```python
from build123d import *

# Parameters (mm, degrees)
F1_DEPTH = 25.4
F3_DEPTH = 25.401
F5_DEPTH = 25.401


with BuildPart() as f1:
    # F0 (on Top) → F1 (new body)
    with BuildSketch(Plane.XY):
        with BuildLine():
            Line((58.851477, 66.675), (0, 66.675))
            Line((0, 66.675), (-69.85, 66.675))
            Line((-69.85, 66.675), (-69.85, 53.975))
            ThreePointArc((-69.85, 53.975), (-71.709872, 49.484872), (-76.2, 47.625))
            Line((-76.2, 47.625), (-88.9, 47.625))
            ThreePointArc((-88.9, 47.625), (-93.390128, 45.765128), (-95.25, 41.275))
            Line((-95.25, 41.275), (-95.25, -79.375))
            ThreePointArc((-95.25, -79.375), (-93.390128, -83.865128), (-88.9, -85.725))
            Line((-88.9, -85.725), (-76.2, -85.725))
            ThreePointArc((-76.2, -85.725), (-71.709872, -83.865128), (-69.85, -79.375))
            Line((-69.85, -79.375), (-69.85, -73.025))
            ThreePointArc((-69.85, -73.025), (-67.990128, -68.534872), (-63.5, -66.675))
            Line((-63.5, -66.675), (0, -66.675))
            Line((0, -66.675), (63.5, -66.675))
            ThreePointArc((63.5, -66.675), (67.990128, -68.534872), (69.85, -73.025))
            Line((69.85, -73.025), (69.85, -79.375))
            ThreePointArc((69.85, -79.375), (71.709872, -83.865128), (76.2, -85.725))
            Line((76.2, -85.725), (88.9, -85.725))
            ThreePointArc((88.9, -85.725), (93.390128, -83.865128), (95.25, -79.375))
            Line((95.25, -79.375), (95.25, 41.275))
            ThreePointArc((95.25, 41.275), (93.390128, 45.765128), (88.9, 47.625))
            Line((88.9, 47.625), (73.516174, 47.625))
            ThreePointArc((73.516174, 47.625), (70.341174, 48.475739), (68.016913, 50.8))
            Line((68.016913, 50.8), (58.851477, 66.675))
        make_face()
        with BuildLine():
            ThreePointArc((-85.725, 31.75), (-82.55, 34.925), (-79.375, 31.75))
            Line((-79.375, 31.75), (-79.375, -69.85))
            ThreePointArc((-79.375, -69.85), (-82.55, -73.025), (-85.725, -69.85))
            Line((-85.725, -69.85), (-85.725, 31.75))
        make_face(mode=Mode.SUBTRACT)
        with BuildLine():
            Line((79.375, -69.85), (79.375, 31.75))
            ThreePointArc((79.375, 31.75), (82.55, 34.925), (85.725, 31.75))
            Line((85.725, 31.75), (85.725, -69.85))
            ThreePointArc((85.725, -69.85), (82.55, -73.025), (79.375, -69.85))
        make_face(mode=Mode.SUBTRACT)
    extrude(amount=F1_DEPTH)

    # F2 (on face) → F3 (cut, through all)
    with BuildSketch(Plane.XY.offset(25.4)):
        Polygon((65.975549, 43.337223), (52.501477, 66.675), (47.738977, 66.675), (62.403674, 41.275), align=None)
    extrude(amount=-F3_DEPTH, mode=Mode.SUBTRACT)

    # F4 (on face) → F5 (cut, through all)
    with BuildSketch(Plane.XY.offset(25.4)):
        Polygon((62.195398, 30.637223), (41.388977, 66.675), (36.626477, 66.675), (58.623523, 28.575), align=None)
        Polygon((62.08142, 11.587223), (30.276477, 66.675), (25.513977, 66.675), (58.509545, 9.525), align=None)
        Polygon((19.163977, 66.675), (14.401477, 66.675), (47.397045, 9.525), (50.96892, 11.587223), align=None)
        Polygon((8.051477, 66.675), (3.288977, 66.675), (36.284545, 9.525), (39.85642, 11.587223), align=None)
        Polygon((-3.061023, 66.675), (-7.823523, 66.675), (25.172045, 9.525), (28.74392, 11.587223), align=None)
        Polygon((-14.173523, 66.675), (-18.936023, 66.675), (14.059545, 9.525), (17.63142, 11.587223), align=None)
        Polygon((-25.286023, 66.675), (-30.048523, 66.675), (2.947045, 9.525), (6.51892, 11.587223), align=None)
        Polygon((-36.398523, 66.675), (-41.161023, 66.675), (-8.165455, 9.525), (-4.59358, 11.587223), align=None)
        Polygon((-47.511023, 66.675), (-52.273523, 66.675), (-19.277955, 9.525), (-15.70608, 11.587223), align=None)
        Polygon((-58.623523, 66.675), (-63.386023, 66.675), (-30.390455, 9.525), (-26.81858, 11.587223), align=None)
        Polygon((-69.736023, 66.675), (-74.498523, 66.675), (-41.502955, 9.525), (-37.93108, 11.587223), align=None)
    extrude(amount=-F5_DEPTH, mode=Mode.SUBTRACT)


solid = f1.part
```
Here's how the part is built. I have some questions about the finished solid (model axes, mm). A direction names the side the tool comes from. Give positions to 0.01 mm unless a question says otherwise; leave off trailing zeros. Loops run counter-clockwise (first coordinate to the right, second up) from the corner with the lowest first, then second, coordinate; pieces in that order, holes last. Notation, with made-up numbers: M 49,14.25 L 67,14.25 A15 ccw 67,43.25 Z; hole C 40.5,65 d3. An arc over 180 degrees is marked long. Put each result on its own line as item: value. Start each with the question number.
(1) I need wall thicknesses on line 1 along X through (y, z) = (-46, 23.5) (3 decimals); line 2 along X through (y, z) = (-73.5, 2.75); line 3 along Y through (x, z) = (29.5, 9.5) (3 decimals). Which ranges of each line are inside material? Lowest first, please. Write a range as [from, to].
(2) I want a section at D-D on z = 10.75. State how many separate pieces and enclosed holes the cut face has, then the cut area to 3 significant figures.
(3) I want a section at A-A on y = -33. Please give me the cut outline in (x, z) (3 decimals), then the cut area to 3 significant figures.
(4) If we mould it in two halves opening along X, with no side actions, what happens to faces 1 (the cylindrical face through (93.439, 45.715, 12.522)), 2 (the flat face through (-11, 66.675, 13)), 3 (the flat face through (54.97, 54.15, 12.88)), 4 (the flat face through (30.67, 38.5, 12.88))? For each: +X half, -X half, draft (parallel to the pull), parting line (faces both ways), or undercut.
(5) For faces 5 (the flat face through (-82, 47.625, 13)), 6 (the flat face through (-1, -66.675, 13)), 7 (the cylindrical face through (-82.48, -73.024, 12.522)), 8 (the flat face through (81, 47.625, 13)), which set-ups out of +Z, -Z, +X, -X, +Y, -Y let a thin tool reach every point of the face, with its end or its side?
(6) I want a section at B-B on x = 82.55. Please give me the cut outline in (y, z) (3 decimals).
(7) I want a section at C-C on x = 22. Please give me the cut outline in (y, z) (3 decimals), then the cut area to 3 significant figures.
(8) Will these pins go through, and if not, where does the flat tip stop? pin 1 Ø8 at (x, z) = (-52, 9) entering from -Y (3 decimals); pin 2 Ø3.5 at (y, z) = (55.5, 11) entering from -X; pin 3 Ø4.5 at (x, z) = (80, 14.5) entering from +Y (3 decimals).
Answer block:
1. line 1: [-95.25, -85.725], [-79.375, 79.375], [85.725, 95.25]
1. line 2: [-95.25, -69.85], [69.85, 95.25]
1. line 3: [-66.675, 21.276], [29.525, 40.524], [48.772, 59.771]
2. separate pieces: 1
2. enclosed holes: 2
2. area: 21,000 mm^2
3. outline: M -95.25,0 L -85.725,0 L -85.725,25.4 L -95.25,25.4 Z; M -79.375,0 L 79.375,0 L 79.375,25.4 L -79.375,25.4 Z; M 85.725,0 L 95.25,0 L 95.25,25.4 L 85.725,25.4 Z
3. area: 4,520 mm^2
4. face 1: +X half
4. face 2: draft
4. face 3: undercut
4. face 4: undercut
5. face 5: +Z, -Z, -X, +Y
5. face 6: +Z, -Z, -Y
5. face 7: +Z, -Z
5. face 8: +Z, -Z, +X, +Y
6. outline: M -85.725,0 L -73.025,0 L -73.025,25.4 L -85.725,25.4 Z; M 34.925,0 L 47.625,0 L 47.625,25.4 L 34.925,25.4 Z
7. outline: M -66.675,0 L 15.019,0 L 15.019,25.4 L -66.675,25.4 Z; M 23.268,0 L 34.267,0 L 34.267,25.4 L 23.268,25.4 Z; M 42.515,0 L 53.514,0 L 53.514,25.4 L 42.515,25.4 Z; M 61.763,0 L 66.675,0 L 66.675,25.4 L 61.763,25.4 Z
7. area: 2,760 mm^2
8. pin 1: y = -66.675
8. pin 2: x = -69.85
8. pin 3: y = 47.625
